For this review, use the dimensioned drawing (mm, ordinates from the lowest corner) and the shaded views. Round coordinates to 2 decimals unless told otherwise and drop trailing zeros. Loops run counter-clockwise (first coordinate to the right, second up) from the corner with the lowest first, then second, coordinate; pieces in that order, holes last. Notation, with made-up numbers: (3.25, 85.5) -> (10.25, 85.5) arc R22 ccw to (10.25, 92.5) -> close; hole circle Ø4 at (32, 40.5). An arc over 180 degrees is marked (long way). Answer as CSV lines item,"result". Start each with the question number.
(1) Take a section at B-B, the plane y = 36.5. State how many separate pieces and enclosed holes the cut face has.
(2) Take a section at A-A, the plane x = 38.1. Write out the cut boundary in (y, z) (1 decimal), and give its area (3 significant figures).
(3) Draft analysis for pull direction Y (two halves, no side actions). For the marked faces 1, 2 and 3, state which applies: +Y half, -Y half, draft (parallel to the pull), parting line (faces both ways), or undercut.
(4) For P1, Ø1, axis at y = 7.5, z = 1, coming from the -X side; P2, Ø1, axis at x = 52, z = 1.5, coming from the -Y side, all flat-tipped, find the tip position at first contact; note any pin that passes through.
(5) Take a section at D-D, the plane y = 5. Write out the cut boundary in (x, z) (1 decimal).
(6) To check wall thickness, follow line 1 (Y direction, x = 19.05, z = 2.2); line 2 (X direction, y = 10, z = 1.9); line 3 (X direction, y = 9, z = 0.5). State the ranges of each line that lie inside material, in increasing order. Write a range as from..to.
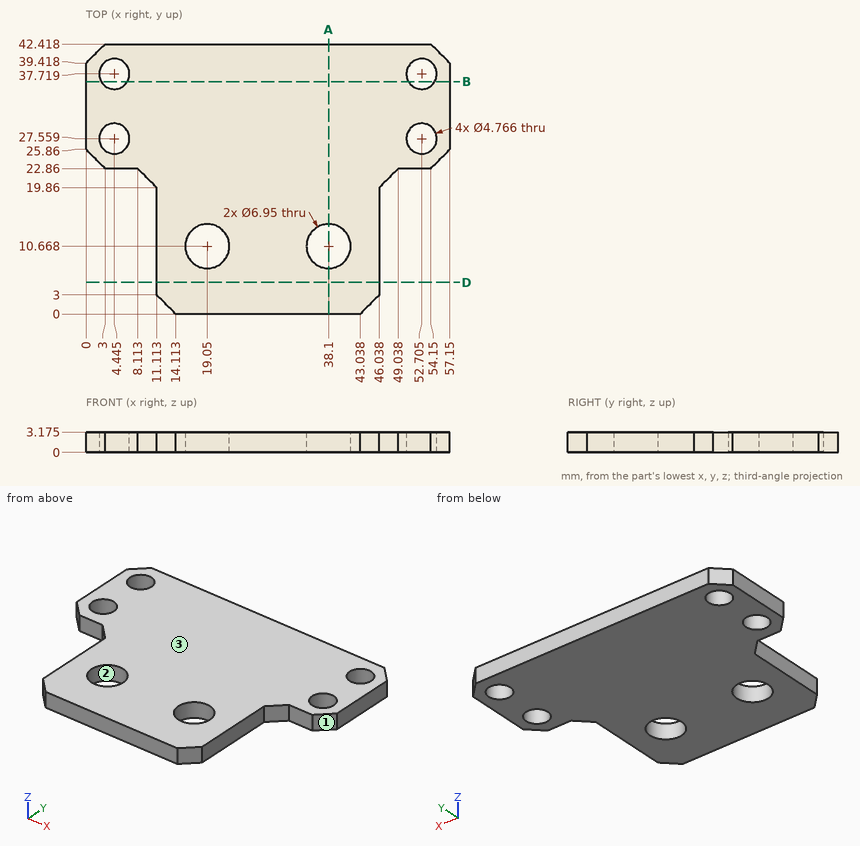
The answers:
1,separate pieces,"3"
1,enclosed holes,"0"
2,outline,"(0, 0) -> (7.2, 0) -> (7.2, 3.2) -> (0, 3.2) -> close; (14.1, 0) -> (42.4, 0) -> (42.4, 3.2) -> (14.1, 3.2) -> close"
2,area,"113 mm²"
3,face 1,"-Y half"
3,face 2,"undercut"
3,face 3,"draft"
4,P1,"x = 11.11"
4,P2,"y = 22.86"
5,outline,"(11.1, 0) -> (46, 0) -> (46, 3.2) -> (11.1, 3.2) -> close"
6,line 1,"0..7.19, 14.14..42.42"
6,line 2,"11.11..15.64, 22.46..34.69, 41.51..46.04"
6,line 3,"11.11..16, 22.1..35.05, 41.15..46.04"
